Study the drawing (mm; zero at the part's minimum x, y, z) and answer. A direction names the side the tool comes from. Round coordinates to 2 decimals unless told otherwise and drop trailing zeros. Write each loop counter-clockwise with the first axis right and the second up, starting at its lowest first coordinate (ties: lowest second). Pieces come first, ordered by that corner, then holes.
(1) The mould has two halves that part along X. Classify the marked faces 4, 5 and 6: +X half, -X half, draft (parallel to the pull), parting line (faces both ways), or undercut.
(2) For the marked faces 1, 2 and 3, determine the directions among +Z, -Z, +X, -X, +Y, -Y from which every point of the face is accessible in a straight line to the end or side of a thin tool.
(3) A cutting plane is placed at B-B, the plane y = 20. Give the vertices of the cut face in (x, z).
(4) A cutting plane is placed at D-D, the plane z = 27.5. Give the vertices of the cut face in (x, y), and give its area (3 significant figures).
(5) A cutting plane is placed at C-C, the plane x = 9. Give the vertices of the cut face in (y, z), and give its area (3 significant figures).
(6) A cutting plane is placed at A-A, the plane x = 22. Give the vertices of the cut face in (y, z), and give its area (3 significant figures).
(7) Each of these flat-tipped pins is pushed along its axis until it touches: pin 1 Ø5 at (y, z) = (18, 7) entering from -X; pin 2 Ø6 at (x, y) = (24.5, 33.5) entering from -Z; pin 3 Ø5 at (x, z) = (15, 4.5) entering from +Y. Where does it stop, or does it pass through?
(8) Find the intervals of material crossed by probe 1 along Y at (x, z) = (38, 8.5); probe 2 along Z at (x, y) = (36, 32); probe 3 along X at (y, z) = (2.5, 3), in increasing order.
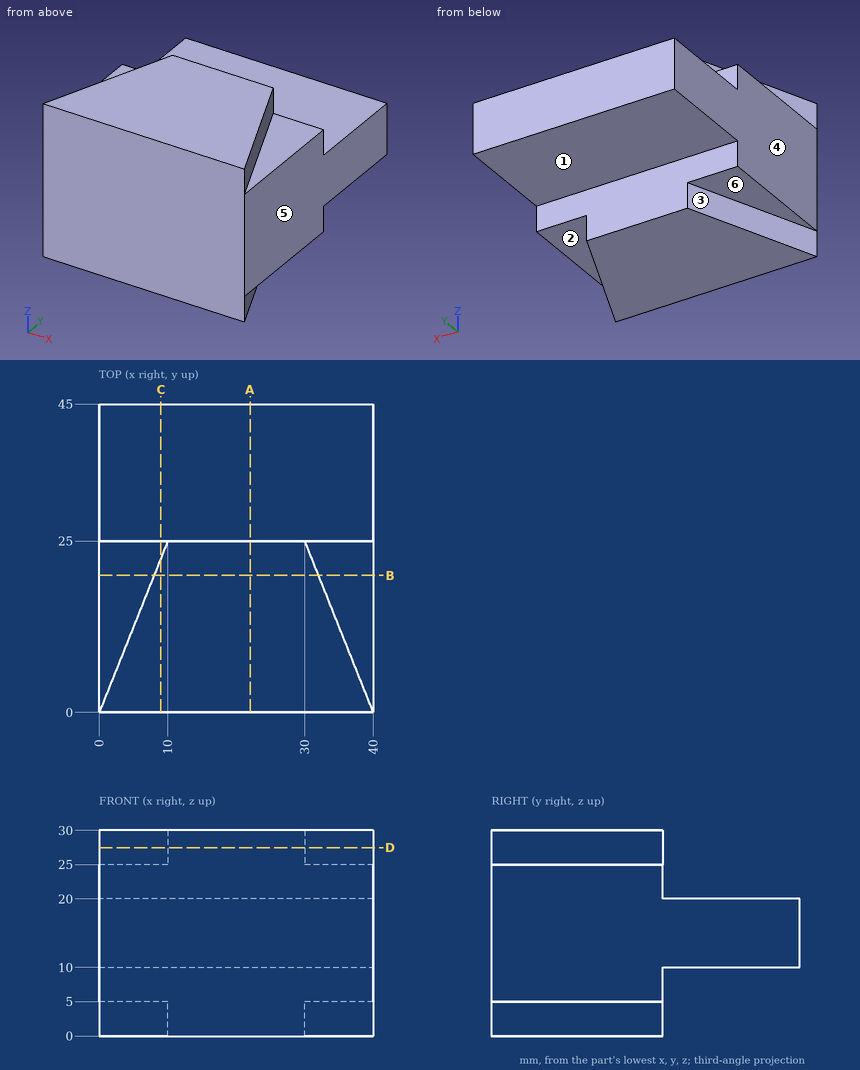
Solutions:
1. face 4: -X half
1. face 5: +X half
1. face 6: draft
2. face 1: -Z, +X, -X, +Y
2. face 2: -Z, +X, +Y
2. face 3: -Z, -X, +Y
3. outline: (0, 5) - (8, 5) - (8, 0) - (32, 0) - (32, 5) - (40, 5) - (40, 25) - (32, 25) - (32, 30) - (8, 30) - (8, 25) - (0, 25) - close
4. outline: (0, 0) - (40, 0) - (30, 25) - (10, 25) - close
4. area: 750 mm2
5. outline: (0, 0) - (22.5, 0) - (22.5, 5) - (25, 5) - (25, 10) - (45, 10) - (45, 20) - (25, 20) - (25, 25) - (22.5, 25) - (22.5, 30) - (0, 30) - close
5. area: 925 mm2
6. outline: (0, 0) - (25, 0) - (25, 10) - (45, 10) - (45, 20) - (25, 20) - (25, 30) - (0, 30) - close
6. area: 950 mm2
7. pin 1: stops at x = 0
7. pin 2: stops at z = 10
7. pin 3: stops at y = 25
8. probe 1: y = 0 to 25
8. probe 2: z = 10 to 20
8. probe 3: x = 1 to 39
